Build history of the part. All positions in model axes, mm. Round coordinates to 2 decimals unless told otherwise and drop trailing zeros. Write each loop counter-clockwise with the first axis right and the second up, starting at its lowest first coordinate (ties: lowest second). Pieces come first, ordered by that corner, then holes. Notation, with made-up numbers: (17.25, -28.5) -> (50.25, -28.5) arc R26 ccw to (50.25, -5.5) -> close; hole circle Ø10 at (26, 66). An arc over 180 degrees is marked (long way). One line per question, with ' | ' between items.
Autodesk Inventor part; units mm, degrees
ref_plane "YZ Plane" through (0, 0, 0) normal (1, 0, 0) x (0, 1, 0)
ref_plane "XZ Plane" through (0, 0, 0) normal (0, 1, 0) x (-1, 0, 0)
ref_plane "XY Plane" through (0, 0, 0) normal (0, 0, 1) x (1, 0, 0)
sketch "Sketch1" plane through (0, 0, 0) normal (0, 0, 1) x (1, 0, 0)
  line L0 (-37.5, 53.5) -> (37.5, 53.5)
  line L1 (37.5, 53.5) -> (37.5, -53.5)
  line L2 (37.5, -53.5) -> (-37.5, -53.5)
  line L3 (-37.5, -53.5) -> (-37.5, 53.5)
  line L4 (-37.5, 53.5) -> (37.5, -53.5) construction
  line L5 (37.5, 53.5) -> (-37.5, -53.5) construction
  line L6 (-25.5, 43.5) -> (-13.5, 43.5)
  line L7 (-8.5, 38.5) -> (-8.5, 7.5)
  line L8 (-13.5, 2.5) -> (-25.5, 2.5)
  line L9 (-30.5, 7.5) -> (-30.5, 38.5)
  line L10 (-30.5, 43.5) -> (-8.5, 2.5) construction
  line L11 (-8.5, 43.5) -> (-30.5, 2.5) construction
  arc A0 (-25.5, 43.5) -> (-30.5, 38.5) centre (-25.5, 38.5) ccw
  arc A1 (-8.5, 38.5) -> (-13.5, 43.5) centre (-13.5, 38.5) ccw
  arc A2 (-13.5, 2.5) -> (-8.5, 7.5) centre (-13.5, 7.5) ccw
  arc A3 (-30.5, 7.5) -> (-25.5, 2.5) centre (-25.5, 7.5) ccw
  line L12 (9.5, 7.5) -> (9.5, 38.5)
  arc A4 (26.5, 2.5) -> (31.5, 7.5) centre (26.5, 7.5) ccw
  arc A5 (14.5, 43.5) -> (9.5, 38.5) centre (14.5, 38.5) ccw
  arc A6 (31.5, 38.5) -> (26.5, 43.5) centre (26.5, 38.5) ccw
  arc A7 (9.5, 7.5) -> (14.5, 2.5) centre (14.5, 7.5) ccw
  line L13 (26.5, 2.5) -> (14.5, 2.5)
  line L14 (31.5, 38.5) -> (31.5, 7.5)
  line L15 (9.5, 43.5) -> (31.5, 2.5) construction
  line L16 (14.5, 43.5) -> (26.5, 43.5)
  line L17 (31.5, 43.5) -> (9.5, 2.5) construction
  line L18 (-30.5, -42.5) -> (-30.5, -11.5)
  arc A8 (-13.5, -47.5) -> (-8.5, -42.5) centre (-13.5, -42.5) ccw
  arc A9 (-25.5, -6.5) -> (-30.5, -11.5) centre (-25.5, -11.5) ccw
  arc A10 (-8.5, -11.5) -> (-13.5, -6.5) centre (-13.5, -11.5) ccw
  arc A11 (-30.5, -42.5) -> (-25.5, -47.5) centre (-25.5, -42.5) ccw
  line L19 (-13.5, -47.5) -> (-25.5, -47.5)
  line L20 (-8.5, -11.5) -> (-8.5, -42.5)
  line L21 (-30.5, -6.5) -> (-8.5, -47.5) construction
  line L22 (-25.5, -6.5) -> (-13.5, -6.5)
  line L23 (-8.5, -6.5) -> (-30.5, -47.5) construction
  line L24 (9.5, -42.5) -> (9.5, -11.5)
  arc A12 (26.5, -47.5) -> (31.5, -42.5) centre (26.5, -42.5) ccw
  arc A13 (14.5, -6.5) -> (9.5, -11.5) centre (14.5, -11.5) ccw
  arc A14 (31.5, -11.5) -> (26.5, -6.5) centre (26.5, -11.5) ccw
  arc A15 (9.5, -42.5) -> (14.5, -47.5) centre (14.5, -42.5) ccw
  line L25 (26.5, -47.5) -> (14.5, -47.5)
  line L26 (31.5, -11.5) -> (31.5, -42.5)
  line L27 (9.5, -6.5) -> (31.5, -47.5) construction
  line L28 (14.5, -6.5) -> (26.5, -6.5)
  line L29 (31.5, -6.5) -> (9.5, -47.5) construction
  line L30 (0, 0) -> (0, 8.3009)
  line L31 (0, 0) -> (4.4939, 0)
  point P0 (-19.5, 23)
  point P1 (20.5, 23)
  point P2 (-19.5, -27)
  point P3 (20.5, -27)
  dimension "d0" = 107
  dimension "d1" = 75
  dimension "d3" = 22
  dimension "d4" = 41
  dimension "d5" = 5
  dimension "d8" = 40
  dimension "d11" = 50
  dimension "d14" = 10
  dimension "d15" = 7
extrude "Plate1" add sketch "Sketch1" along normal blind 1
sketch "Sketch2" plane through (0, 0, 1) normal (0, 0, 1) x (1, 0, 0)
  line L0 (37.5, 53.5) -> (37.5, -53.5)
  line L1 (-37.5, -53.5) -> (-37.5, 53.5)
  line L2 (-47.5, 5) -> (-37.5, 5)
  line L3 (-37.5, 5) -> (-37.5, -5)
  line L4 (-37.5, -5) -> (-47.5, -5)
  line L5 (-47.5, -5) -> (-47.5, 5)
  line L6 (-47.5, 5) -> (-37.5, -5) construction
  line L7 (-37.5, 5) -> (-47.5, -5) construction
  line L8 (-37.5, 53.5) -> (37.5, 53.5)
  line L9 (-5, 63.5) -> (5, 63.5)
  line L10 (5, 63.5) -> (5, 53.5)
  line L11 (5, 53.5) -> (-5, 53.5)
  line L12 (-5, 53.5) -> (-5, 63.5)
  line L13 (-5, 63.5) -> (5, 53.5) construction
  line L14 (5, 63.5) -> (-5, 53.5) construction
  line L15 (0, 0) -> (10.0151, 0)
  line L16 (-5, -63.5) -> (5, -63.5)
  line L17 (5, -63.5) -> (5, -53.5)
  line L18 (5, -53.5) -> (-5, -53.5)
  line L19 (-5, -53.5) -> (-5, -63.5)
  line L20 (-5, -63.5) -> (5, -53.5) construction
  line L21 (5, -63.5) -> (-5, -53.5) construction
  circle A0 centre (0, 59.5) radius 1.6
  circle A1 centre (-43.5, 0) radius 1.6
  circle A2 centre (0, -59.5) radius 1.6
  point P0 (-42.5, 0)
  point P1 (0, 58.5)
  point P2 (0, -58.5)
  point P3 (37.5, 38.5)
  dimension "d23" = 10
  dimension "d24" = 10
  dimension "d27" = 10
  dimension "d28" = 10
  dimension "d43" = 3.2
  dimension "d44" = 3.2
  dimension "d45" = 4
  dimension "d46" = 4
sheet face with bend "Face2" sketch "Sketch2" thickness 1 toward (0, 0, -1) bend radius 1
bend "Bend1"
sketch "Sketch3" plane through (0, 0, 1) normal (0, 0, 1) x (1, 0, 0)
  circle A0 centre (2.5, -18.5) radius 1.6
  line L0 (2.5, -18.5) -> (11.3604, -18.5)
  line L1 (2.5, -18.5) -> (2.5, -34.5603)
  circle A1 centre (34.5, -18.5) radius 1.6
  circle A2 centre (2.5, -50.5) radius 1.6
  circle A3 centre (34.5, -50.5) radius 1.6
  line L2 (37.5, 53.5) -> (37.5, -53.5)
  line L3 (37.5, -53.5) -> (5, -53.5)
  point P0 (0, 0)
  dimension "d48" = 3.2
  dimension "d51" = 32
  dimension "d54" = 32
  dimension "d57" = 35
  dimension "d58" = 35
extrude "Cut1" cut sketch "Sketch3" against normal blind 1
equation "\"d59\" = 厚度"
equation "\"d2\" = 厚度"
equation "\"d37\" = 折彎半徑"
equation "\"d38\" = 折彎離隙寬度"
equation "\"d40\" = 最小剩餘"
equation "\"d39\" = 折彎離隙深度"
equation "\"d41\" = 轉移半徑"
equation "\"折彎半徑\" = 厚度"
equation "\"折彎離隙寬度\" = 厚度"
equation "\"折彎離隙深度\" = 0.5 * 厚度"
equation "\"轉角離隙大小\" = 4 * 厚度"
equation "\"最小剩餘\" = 2 * 厚度"
equation "\"轉移半徑\" = 折彎半徑"
equation "\"Jacobi半徑大小\" = 折彎半徑"
equation "\"間隙大小\" = 厚度"
properties part number "PCB_board_box_right" material "Aluminum"
(1) Slice it at D-D (z = 0.6). State how many separate pieces and enclosed holes the cut face has, then the cut area to 3 significant figures.
Calculated:
separate pieces: 1 | enclosed holes: 11 | area: 4,750 mm2
(2) Drop flat-ended pins along their axis: pin 1 (4 mm diameter, centred on x = 34.5, y = -18.5, fed in from +Z); pin 2 (0.5 mm diameter, centred on x = 15.5, z = 0.5, fed in from -Y); pin 3 (0.5 mm diameter, centred on y = 25.5, z = 0.5, fed in from -X); pin 4 (0.5 mm diameter, centred on y = -60, z = 0.5, fed in from -X). Give the stop position or say it passes through.
Calculated:
pin 1: z = 1 | pin 2: y = -53.5 | pin 3: x = -37.5 | pin 4: x = -5
(3) Slice it at A-A (x = 19). Write the cut outline in (y, z).
Calculated:
outline: (-53.5, 0) -> (-47.5, 0) -> (-47.5, 1) -> (-53.5, 1) -> close; (-6.5, 0) -> (2.5, 0) -> (2.5, 1) -> (-6.5, 1) -> close; (43.5, 0) -> (53.5, 0) -> (53.5, 1) -> (43.5, 1) -> close
(4) Mould opens along X. For faces 1 (the cylindrical face through (-9.93, -46, 0.49)), 2 (the flat face through (4, 1, 1)) say: pulls with the +X half, pulls with the -X half, needs draft (parallel to the pull), parting line crosses it, or undercut.
Calculated:
face 1: undercut | face 2: needs draft
(5) Wall check: line 1 (X direction, y = 17.5, z = 0.35); line 2 (Y direction, x = 22, z = 0.95); line 3 (Y direction, x = 2.5, z = 0.7). Give the ranges that are in metal, low to high. Write a range as from..to.
Calculated:
line 1: -37.5..-30.5, -8.5..9.5, 31.5..37.5 | line 2: -53.5..-47.5, -6.5..2.5, 43.5..53.5 | line 3: -63.5..-52.1, -48.9..-20.1, -16.9..63.5
(6) Slice it at B-B (y = 59.5). Write the cut outline in (x, z), then the cut area to 3 significant figures.
Calculated:
outline: (-5, 0) -> (-1.6, 0) -> (-1.6, 1) -> (-5, 1) -> close; (1.6, 0) -> (5, 0) -> (5, 1) -> (1.6, 1) -> close | area: 6.80 mm2
